For this review, take the finished solid that the model builds, in its own axes (mm). A direction names the side the tool comes from. Give positions to 0.01 mm unless a question says otherwise; leave off trailing zeros. Loops run counter-clockwise (first coordinate to the right, second up) from the corner with the lowest first, then second, coordinate; pieces in that order, holes last.
```python
from build123d import *

# Parameters (mm, degrees)
BOSS_EXTRUDE2_DEPTH      = 13
CUT_EXTRUDE6_DEPTH       = 43.108996013
CUT_EXTRUDE7_DEPTH       = 43.108996013
CUT_EXTRUDE8_DEPTH       = 13
SKETCH7_R                = 4.2
CUT_EXTRUDE9_DEPTH       = 30
BOSS_EXTRUDE3_DEPTH      = 10
CUT_EXTRUDE10_DEPTH      = 1
SKETCH13_R               = 4.2
BOSS_EXTRUDE4_DEPTH      = 20.09
SKETCH17_W               = 13
SKETCH17_H               = 15.432451
BOSS_EXTRUDE5_DEPTH      = 10.6
CHAMFER1_SIZE            = 10.6
SKETCH12_R               = 3
CUT_EXTRUDE11_DEPTH      = 77.770333281
CUT_EXTRUDE12_START      = -6.148636
CUT_EXTRUDE12_DEPTH      = 5.3
FILLET2_R                = 2
SKETCH25_W               = 86.308607618
SKETCH25_H               = 69.103285455
CUT_EXTRUDE13_DEPTH      = 0.00151491
CUT_EXTRUDE14_DEPTH      = 58.985456967
CUT_EXTRUDE15_REACH      = 89.237
CUT_EXTRUDE15_END_RADIUS = 11.5
SKETCH27_W               = 4
SKETCH27_H               = 8
SKETCH28_W               = 26.149590075
SKETCH28_H               = 8.463351347
CUT_EXTRUDE16_DEPTH      = 3
FILLET9_R                = 2
SKETCH34_R               = 4.2
BOSS_EXTRUDE7_DEPTH      = 5
CUT_EXTRUDE22_START      = -13
CUT_EXTRUDE22_DEPTH      = 13
CUT_EXTRUDE23_DEPTH      = 58.985456967
CUT_EXTRUDE24_START      = -1
CUT_EXTRUDE24_DEPTH      = 10
CHAMFER2_SIZE            = 0.5


# Read off the part's stored shape, not the designer's step: Cut-Extrude22
with BuildPart() as part:
    # Sketch1 → Boss-Extrude2 (new body)
    with BuildSketch(Plane(origin=(0, 0, 0), x_dir=(1, 0, 0), z_dir=(0, 1, 0))):
        Polygon((-2.969848481, 26.728636329), (-6.906313813, 26.728636329), (-29.828636329, 3.806313813), (-29.828636329, -2.969848481), (-6.069848481, -26.728636329), (-2.969848481, -26.728636329), (2.969848481, -26.728636329), (29.69848481, -26.728636329), (29.69848481, 26.728636329), (2.969848481, 26.728636329), align=None)
    extrude(amount=BOSS_EXTRUDE2_DEPTH)

    # Sketch1<8> → Cut-Extrude6 (cut, through all)
    with BuildSketch(Plane(origin=(0, 0, 0), x_dir=(1, 0, 0), z_dir=(0, 1, 0))):
        with BuildLine():
            Line((-23.14, -1.55), (-20.04, -1.55))
            ThreePointArc((-20.04, -1.55), (-18.49, 0), (-20.04, 1.55))
            Line((-20.04, 1.55), (-23.14, 1.55))
            ThreePointArc((-23.14, 1.55), (-24.69, 0), (-23.14, -1.55))
        make_face()
    extrude(amount=CUT_EXTRUDE6_DEPTH, mode=Mode.SUBTRACT)

    # Sketch1<9> → Cut-Extrude7 (cut, through all)
    with BuildSketch(Plane(origin=(0, 0, 0), x_dir=(1, 0, 0), z_dir=(0, 1, 0))):
        with BuildLine():
            Line((9.28999972, -8.505433812), (9.28999972, 8.505433812))
            ThreePointArc((9.28999972, 8.505433812), (5.69954884, 10.725261974), (1.55, 11.5))
            Line((1.55, 11.5), (-1.55, 11.5))
            ThreePointArc((-1.55, 11.5), (-13.05, 0), (-1.55, -11.5))
            Line((-1.55, -11.5), (1.55, -11.5))
            ThreePointArc((1.55, -11.5), (5.69954884, -10.725261974), (9.28999972, -8.505433812))
        make_face()
        with BuildLine():
            ThreePointArc((9.28999972, -8.505433812), (13.05, 0), (9.28999972, 8.505433812))
            Line((9.28999972, 8.505433812), (9.28999972, -8.505433812))
        make_face()
    extrude(amount=CUT_EXTRUDE7_DEPTH, mode=Mode.SUBTRACT)

    # Sketch1<11> → Cut-Extrude8 (cut)
    with BuildSketch(Plane(origin=(0, 0, 0), x_dir=(1, 0, 0), z_dir=(0, 1, 0))):
        with BuildLine():
            Line((23.139619127, 1.551521906), (20.03999972, 1.550761))
            ThreePointArc((20.03999972, 1.550761), (18.48961936, 0), (20.03999972, -1.550761))
            Line((20.03999972, -1.550761), (23.14, -1.551521999))
            ThreePointArc((23.14, -1.551521999), (24.691521964, 0.000190413), (23.139619127, 1.551521906))
        make_face()
        with BuildLine():
            ThreePointArc((21.589619103, -0.059493857), (21.588478024, -1.2e-08), (21.589619104, 0.059493833))
            ThreePointArc((21.589619104, 0.059493833), (21.590760744, -1.2e-08), (21.589619103, -0.059493857))
        make_face(mode=Mode.SUBTRACT)
    extrude(amount=CUT_EXTRUDE8_DEPTH, mode=Mode.SUBTRACT)


with BuildPart() as cut_extrude8_piece_1:
    # of the separate pieces the step leaves, piece 1, a body of its own (cut_extrude8_pieces)
    add(part.part.solids().sort_by_distance((-6.906313813, 0, -26.728636329))[0])

    # Sketch7 → Cut-Extrude9 (cut)
    with BuildSketch(Plane(origin=(29.69848481, 0, 0), x_dir=(0, 0, -1), z_dir=(1, 0, 0))):
        with Locations((-20, 6.5)):
            Circle(SKETCH7_R)
        with Locations((20, 6.5)):
            Circle(SKETCH7_R)
    extrude(amount=-CUT_EXTRUDE9_DEPTH, mode=Mode.SUBTRACT)

    # Sketch9 → Boss-Extrude3 (add)
    with BuildSketch(Plane.XY.offset(26.728636329)):
        with BuildLine():
            Line((-3.11848537, 13), (29.69848481, 13))
            Line((29.69848481, 13), (20.745211893, 22.464823228))
            Line((20.745211893, 22.464823228), (16.754822948, 22.464823228))
            ThreePointArc((16.754822948, 22.464823228), (13.28999972, 14.1), (9.825176492, 22.464823228))
            Line((9.825176492, 22.464823228), (5.834787547, 22.464823228))
            Line((5.834787547, 22.464823228), (-3.11848537, 13))
        make_face()
    boss_extrude3 = extrude(amount=-BOSS_EXTRUDE3_DEPTH)

    # Sketch10 → Cut-Extrude10 (cut)
    with BuildSketch(Plane.XY.offset(24.728636329)):
        with BuildLine():
            Line((6.93999972, 19), (6.93999972, 29.430631577))
            Line((6.93999972, 29.430631577), (19.63999972, 29.430631577))
            Line((19.63999972, 29.430631577), (19.63999972, 19))
            ThreePointArc((19.63999972, 19), (13.28999972, 12.65), (6.93999972, 19))
        make_face()
    cut_extrude10 = extrude(amount=-CUT_EXTRUDE10_DEPTH, mode=Mode.SUBTRACT)

    # Mirror1: Boss-Extrude3, Cut-Extrude10 across plane
    add(boss_extrude3.mirror(Plane.XY))
    add(cut_extrude10.mirror(Plane.XY), mode=Mode.SUBTRACT)

    # Sketch13 → Boss-Extrude4 (add)
    with BuildSketch(Plane(origin=(29.69848481, 0, 0), x_dir=(0, 0, -1), z_dir=(1, 0, 0))):
        Polygon((-26.728636329, 0), (26.728636329, 0), (26.728636329, 13), (16.728636329, 13), (-16.728636329, 13), (-26.728636329, 13), align=None)
        with Locations((-20, 6.5)):
            Circle(SKETCH13_R, mode=Mode.SUBTRACT)
        with Locations((20, 6.5)):
            Circle(SKETCH13_R, mode=Mode.SUBTRACT)
    extrude(amount=BOSS_EXTRUDE4_DEPTH)

    # Sketch17 → Boss-Extrude5 (add)
    with BuildSketch(Plane(origin=(0, 13, 0), x_dir=(1, 0, 0), z_dir=(0, 1, 0))):
        with Locations((43.28999972, 0)):
            Rectangle(SKETCH17_W, SKETCH17_H)
    extrude(amount=BOSS_EXTRUDE5_DEPTH)

    # Chamfer1
    # the kernel refuses this chamfer: 10.6 mm, written as the material it adds along each edge
    with BuildSketch(Plane(origin=(49.78848481, 13, 7.7162255), x_dir=(0, -0.027495876610586376, 0.9996219169112966), z_dir=(-1, 0, 0)), Plane(origin=(36.78999972, 13, -7.7162255), x_dir=(0, -0.02749587661058638, -0.9996219169112966), z_dir=(1, 0, 0))) as chamfer1_piece_1:
        Polygon((CHAMFER1_SIZE * 0.999621916911, CHAMFER1_SIZE * 0.0274958766106), (-CHAMFER1_SIZE * 0.0274958766106, CHAMFER1_SIZE * 0.999621916911), (0, 0), align=None)
    extrude(amount=12.99848509)

    # Sketch12 → Cut-Extrude11 (cut, through all)
    with BuildSketch(Plane.XY.offset(26.728636329)):
        with Locations(Location((43.28999972, 19, 0), (0, 0, 270))):
            Circle(SKETCH12_R)
    extrude(amount=-CUT_EXTRUDE11_DEPTH, mode=Mode.SUBTRACT)

    # Sketch24 → Cut-Extrude12 (cut)
    with BuildSketch(Plane.XY.offset(6.148636329).offset(CUT_EXTRUDE12_START)):
        Polygon((47.273716577, 23.6), (47.273716577, 21.3), (47.273716577, 16.7), (43.28999972, 14.4), (39.306282862, 16.7), (39.306282862, 21.3), (39.306282862, 23.6), align=None)
    cut_extrude12 = extrude(amount=-CUT_EXTRUDE12_DEPTH, mode=Mode.SUBTRACT)

    # Fillet2
    fillet2_edges = [cut_extrude8_piece_1.edges().sort_by_distance(p)[0] for p in [
        (49.78848481, 6.5, 26.728636329),
        (49.78848481, 6.5, -26.728636329),
    ]]
    fillet(fillet2_edges, radius=FILLET2_R)

    # Sketch25 → Cut-Extrude13 (cut)
    with BuildSketch(Plane(origin=(49.78999972, 0, 0), x_dir=(0, 0, -1), z_dir=(1, 0, 0))):
        with Locations((0, 8.901936044)):
            Rectangle(SKETCH25_W, SKETCH25_H)
    extrude(amount=-CUT_EXTRUDE13_DEPTH, mode=Mode.SUBTRACT)

    # Cut-Extrude15: up to this cylinder (the profile starts outside it)
    cut_extrude15_end = Plane(origin=(1.55, 6.5, 0), z_dir=(0, -1, 0)) * Cylinder(CUT_EXTRUDE15_END_RADIUS, 202.474, mode=Mode.PRIVATE)
    # Sketch27 → Cut-Extrude15 (cut, up to the surface)
    with BuildSketch(Plane(origin=(49.78848481, 0, 0), x_dir=(0, 0, -1), z_dir=(1, 0, 0)), mode=Mode.PRIVATE) as cut_extrude15_sk1:
        with Locations((-5.3, 6.5)):
            Rectangle(SKETCH27_W, SKETCH27_H)
    cut_extrude15_tool1 = extrude(cut_extrude15_sk1.sketch, amount=-CUT_EXTRUDE15_REACH, mode=Mode.PRIVATE) - cut_extrude15_end
    cut_extrude15 = cut_extrude15_tool1.solids().sort_by_distance((49.788485, 6.5, 5.3))[0]
    add(cut_extrude15, mode=Mode.SUBTRACT)

    # Mirror2: Cut-Extrude15 across plane
    add(cut_extrude15.mirror(Plane.XY), mode=Mode.SUBTRACT)

    # Mirror3: Cut-Extrude12 across plane
    add(cut_extrude12.mirror(Plane.XY), mode=Mode.SUBTRACT)

    # Sketch28 → Cut-Extrude16 (cut)
    with BuildSketch(Plane.XY.offset(26.728636329)):
        with Locations((11.690030011, 23.231675673)):
            Rectangle(SKETCH28_W, SKETCH28_H)
    cut_extrude16 = extrude(amount=-CUT_EXTRUDE16_DEPTH, mode=Mode.SUBTRACT)

    # Mirror4: Cut-Extrude16 across plane
    add(cut_extrude16.mirror(Plane.XY), mode=Mode.SUBTRACT)

    # Fillet9
    fillet9_edges = [cut_extrude8_piece_1.edges().sort_by_distance(p)[0] for p in [
        (-6.906313813, 6.5, -26.728636329),
        (-29.828636329, 6.5, -3.806313813),
        (-29.828636329, 6.5, 2.969848481),
    ]]
    fillet(fillet9_edges, radius=FILLET9_R)

    # Sketch34 → Boss-Extrude7 (add)
    with BuildSketch(Plane(origin=(-0.30151519, 0, 0), x_dir=(0, 0, -1), z_dir=(1, 0, 0))):
        with Locations((-20, 6.5)):
            Circle(SKETCH34_R)
        with Locations((20, 6.5)):
            Circle(SKETCH34_R)
    extrude(amount=BOSS_EXTRUDE7_DEPTH)

    # Cut-Extrude22 outline → Cut-Extrude22 (cut)
    with BuildSketch(Plane(origin=(0, 13, 0), x_dir=(1, 0, 0), z_dir=(0, 1, 0)).offset(CUT_EXTRUDE22_START)):
        with BuildLine():
            ThreePointArc((-20.04, 1.55), (-18.49, 0), (-20.04, -1.55))
            Line((-20.04, -1.55), (-19.04, -1.55))
            ThreePointArc((-19.04, -1.55), (-17.49, 0), (-19.04, 1.55))
            Line((-19.04, 1.55), (-20.04, 1.55))
        make_face()
        with BuildLine():
            Line((24.139625451, 1.551521906), (23.14, 1.551521953))
            ThreePointArc((23.14, 1.551521953), (24.691521976, -2.3e-08), (23.14, -1.551521999))
            Line((23.14, -1.551521999), (24.139751204, -1.551521977))
            ThreePointArc((24.139751204, -1.551521977), (25.691147394, 6.2838e-05), (24.139625451, 1.551521906))
        make_face()
    extrude(amount=CUT_EXTRUDE22_DEPTH, mode=Mode.SUBTRACT)

    # Sketch38 → Cut-Extrude23 (cut, through all)
    with BuildSketch(Plane(origin=(0, 13, 0), x_dir=(1, 0, 0), z_dir=(0, 1, 0))):
        with BuildLine():
            ThreePointArc((1.55, 11.5), (13.05, 0), (1.55, -11.5))
            Line((1.55, -11.5), (2.55, -11.5))
            ThreePointArc((2.55, -11.5), (14.05, 0), (2.55, 11.5))
            Line((2.55, 11.5), (1.55, 11.5))
        make_face()
    extrude(amount=-CUT_EXTRUDE23_DEPTH, mode=Mode.SUBTRACT)

    # Sketch39 → Cut-Extrude24 (cut)
    with BuildSketch(Plane(origin=(0, 2.5, 0), x_dir=(1, 0, 0), z_dir=(0, 1, 0)).offset(CUT_EXTRUDE24_START)):
        with BuildLine():
            Line((47.78848481, 7.3), (13.906055653, 7.3))
            ThreePointArc((13.906055653, 7.3), (14.935796911, 5.370478086), (15.640454538, 3.3))
            Line((15.640454538, 3.3), (47.78848481, 3.3))
            Line((47.78848481, 3.3), (47.78848481, 7.3))
        make_face()
        with BuildLine():
            Line((13.906055653, -7.3), (47.78848481, -7.3))
            Line((47.78848481, -7.3), (47.78848481, -3.3))
            Line((47.78848481, -3.3), (15.640454538, -3.3))
            ThreePointArc((15.640454538, -3.3), (14.935796911, -5.370478086), (13.906055653, -7.3))
        make_face()
    extrude(amount=CUT_EXTRUDE24_DEPTH, mode=Mode.SUBTRACT)

    # Chamfer2
    chamfer2_edges = [cut_extrude8_piece_1.edges().sort_by_distance(p)[0] for p in [
        (0.5, 0, 11.5),
        (-13.05, 0, 0),
        (-24.69, 0, 0),
        (-21.09, 0, -1.55),
        (21.58999986, 0, 1.551141499),
        (18.48961936, 0, 0),
        (-17.49, 0, 0),
        (23.139809563, 0, -1.551521941),
        (25.691147394, 0, -6.2838e-05),
        (23.639875602, 0, 1.551521988),
        (23.639812726, 0, -1.55152193),
        (14.05, 0, 0),
        (-21.09, 0, 1.55),
        (0.5, 0, -11.5),
        (21.589809423, 0, -1.551141453),
    ]]
    chamfer(chamfer2_edges, length=CHAMFER2_SIZE)


with BuildPart() as cut_extrude8_piece_2:
    # of the separate pieces the step leaves, piece 2, a body of its own (cut_extrude8_pieces)
    add(part.part.solids().sort_by_distance((21.589619104, 0, -0.059493833))[0])

    # Sketch26 → Cut-Extrude14 (cut, through all)
    with BuildSketch(Plane(origin=(0, 13, 0), x_dir=(1, 0, 0), z_dir=(0, 1, 0))):
        with BuildLine():
            ThreePointArc((21.589619104, 0.059493833), (21.588478024, -1.2e-08), (21.589619103, -0.059493857))
            ThreePointArc((21.589619103, -0.059493857), (21.590760744, -1.2e-08), (21.589619104, 0.059493833))
        make_face()
    extrude(amount=-CUT_EXTRUDE14_DEPTH, mode=Mode.SUBTRACT)


solid = cut_extrude8_piece_1.part
```
Item 1: Take a section at A-A on z = 0. State how many separate pieces and enclosed holes the cut face has, and give its area (3 significant figures).
Answer:
separate pieces: 4
enclosed holes: 0
area: 568 mm2
Item 2: Take a section at D-D on z = 22. Give the boundary of the cut face in (x, y), and give its area (3 significant figures).
Answer:
outline: (-10.8, 0) - (49.79, 0) - (49.79, 2.81) - (4.7, 2.81) - (4.7, 10.19) - (49.79, 10.19) - (49.79, 13) - (29.7, 13) - (20.75, 22.46) - (16.75, 22.46) arc R4.9 cw (long way) to (9.83, 22.46) - (5.83, 22.46) - (-3.12, 13) - (-10.8, 13) - close
area: 612 mm2
Item 3: Take a section at C-C on z = -20. Give the boundary of the cut face in (x, y).
Answer:
outline: (-13.63, 0) - (49.79, 0) - (49.79, 2.3) - (4.7, 2.3) - (4.7, 10.7) - (49.79, 10.7) - (49.79, 13) - (29.7, 13) - (20.75, 22.46) - (16.75, 22.46) arc R4.9 cw (long way) to (9.83, 22.46) - (5.83, 22.46) - (-3.12, 13) - (-13.63, 13) - close
Item 4: Tool access review of faces 4 (the cylindrical face through (-13.047, 6.662, -0.253)), 5 (the conical face through (-24.825, 0.365, -0.037)), 6 (the cylindrical face through (14.95, 1.99, 5.34)): name each direction out of +Z, -Z, +X, -X, +Y, -Y from which nothing blocks a thin tool from reaching the whole face with its end or side.
Answer:
face 4: +Y, -Y
face 5: -Y
face 6: none
Item 5: Clearance check with flat-ended pins moving along their axes: pin 1 Ø6 at (x, z) = (-12, -5) entering from +Y; pin 2 Ø1 at (y, z) = (20, -12.5) entering from +X; pin 3 Ø7 at (x, y) = (12, 16) entering from +Z; pin 4 Ø4.5 at (x, z) = (19, 21) entering from +Y. State where each tip first meets the part, or that it passes through.
Answer:
pin 1: stops at y = 13
pin 2: passes through
pin 3: stops at z = 26.73
pin 4: stops at y = 22.46
Item 6: The part is to be moulded in two halves that separate along Z. For faces 1 (the cylindrical face through (49.218, 6.591, -26.127)), 2 (the conical face through (-17.355, 0.365, 0.037)), 3 (the flat face through (1.42, 17.8, -21.8)), say which applies: released by +Z, released by -Z, zero draft, split by the parting line, or undercut.
Answer:
face 1: released by -Z
face 2: undercut
face 3: zero draft
Item 7: For L1, parallel to X at y = 19, z = -20.75; L2, parallel to X at y = 19, z = 7.5; L3, parallel to X at y = 2, z = 4, list the stretches that pass through material, from the lowest coordinate up.
Answer:
L1: x = 2.56 to 8.39, 18.19 to 24.02
L2: x = 36.79 to 40.29, 46.29 to 49.79
L3: x = -28.8 to -12.33, 13.33 to 15.44, 47.79 to 49.79
